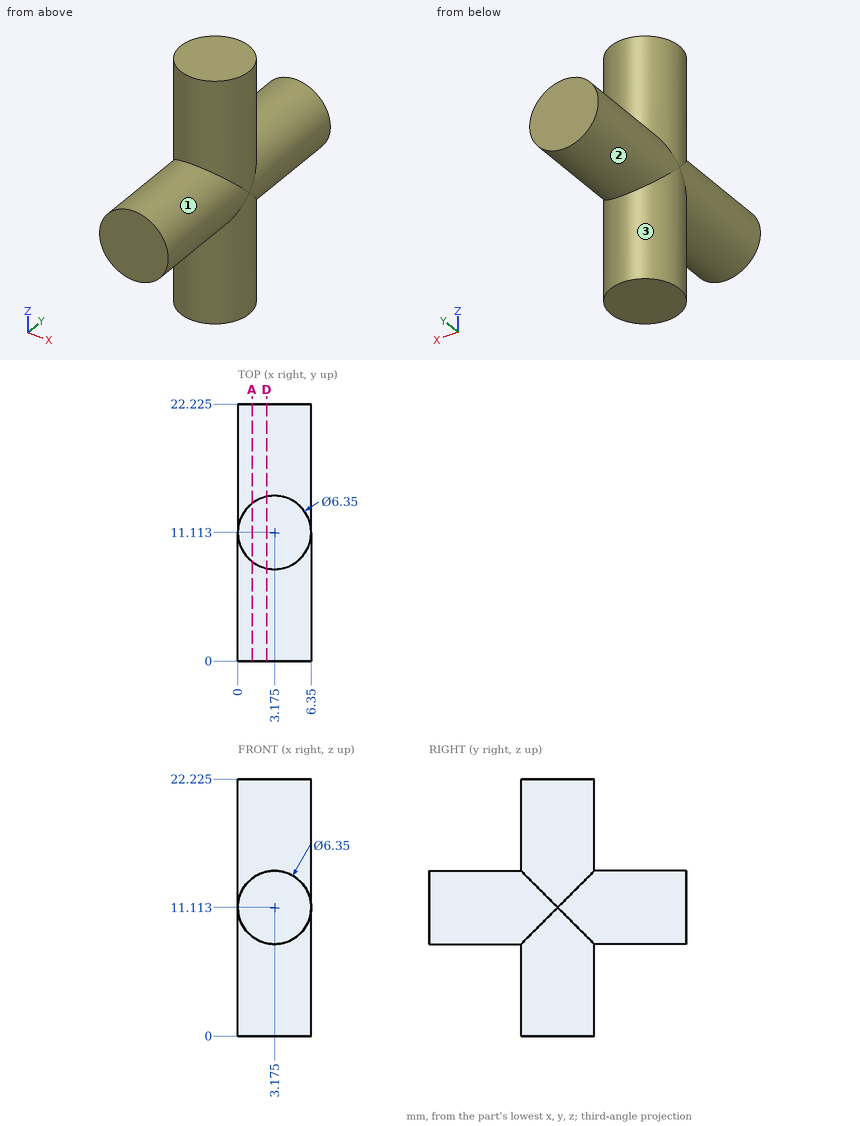
Study the drawing (mm; zero at the part's minimum x, y, z) and answer. A direction names the side the tool comes from. Round coordinates to 2 decimals unless told otherwise and drop trailing zeros. Write each loop counter-clockwise with the first axis right and the second up, starting at its lowest first coordinate (ties: lowest second). Pieces come first, ordered by that corner, then holes. Notation, with made-up numbers: (3, 76.5) - (26, 76.5) arc R27 cw to (26, 111.5) - close; hole circle Ø4 at (-33, -3.5). An arc over 180 degrees is marked (long way). Use a Markdown table: item, result. Add a question column.
1. Consider line 1 (Y direction, x = 0.5, z = 19) (1 decimal); line 2 (Z direction, x = 2.5, y = 3.25) (1 decimal); line 3 (X direction, y = 5.25, z = 9.75). Determine where each line is inside the solid, lowest interval first.
2. The part is cut by section A-A (x = 1.25). Write down the section's boundary in (y, z) (1 decimal), and give its area (3 significant figures).
3. Flat-ended cylindrical pins translate along their axes: P1, Ø1, axis at x = 2.5, y = 3.5, coming from the +Z side; P2, Ø3, axis at x = 0.5, y = 6.5, coming from the +Z side; P3, Ø4, axis at y = 15.5, z = 10, coming from the -X side; P4, Ø3, axis at x = 4.5, z = 4.5, coming from the -Y side. Find the tip coordinate at first contact, or state that the pin passes through.
4. The part is cut by section D-D (x = 2.5). Write down the section's boundary in (y, z) (1 decimal), and give its area (3 significant figures).
5. A tool of negligible diameter and unlimited length cuts with its end or side. For the marked faces 1, 2 and 3, from which of +Z, -Z, +X, -X, +Y, -Y can it reach the whole face along a straight path? Write none if from no direction.
Reported:
| question | item | result |
|---|---|---|
| 1 | line 1 | 9.4 to 12.8 |
| 1 | line 2 | 8 to 14.2 |
| 1 | line 3 | 0.31 to 6.04 |
| 2 | outline | (0, 8.6) - (8.6, 8.6) - (8.6, 0) - (13.6, 0) - (13.6, 8.6) - (22.2, 8.6) - (22.2, 13.6) - (13.6, 13.6) - (13.6, 22.2) - (8.6, 22.2) - (8.6, 13.6) - (0, 13.6) - close |
| 2 | area | 199 mm^2 |
| 3 | P1 | z = 14.28 |
| 3 | P2 | z = 14.06 |
| 3 | P3 | x = 0 |
| 3 | P4 | y = 7.94 |
| 4 | outline | (0, 8) - (8, 8) - (8, 0) - (14.2, 0) - (14.2, 8) - (22.2, 8) - (22.2, 14.2) - (14.2, 14.2) - (14.2, 22.2) - (8, 22.2) - (8, 14.2) - (0, 14.2) - close |
| 4 | area | 237 mm^2 |
| 5 | face 1 | -Y |
| 5 | face 2 | +Y |
| 5 | face 3 | -Z |
